For this review, use the dimensioned drawing (mm, ordinates from the lowest corner) and the shaded views. A direction names the side the tool comes from. Coordinates: 2 decimals unless noted, no trailing zeros. Loops run counter-clockwise (first coordinate to the right, second up) from the corner with the lowest first, then second, coordinate; pieces in that order, holes last. Notation, with made-up numbers: M 67,-39.5 L 77,-39.5 A24 ccw 77,-27.5 Z; hole C -38,-3 d11. An arc over 180 degrees is marked long. Use CSV: the item, a comma, the result in double quotes. Start each with the question number.
1. For L1, parallel to X at y = 1, z = 13; L2, parallel to Z at x = 12.75, y = 3.5; L3, parallel to Y at x = 13.75, z = 12.5, list the stretches that pass through material, from the lowest coordinate up.
2. Add section D-D, the plane y = 7.75. Write out the cut boundary in (x, z).
3. Add section B-B, the plane z = 9.75. Write out the cut boundary in (x, y).
4. Add section C-C, the plane x = 12.7. Write out the cut boundary in (y, z).
5. Clearance check with flat-ended pins moving along their axes: P1, Ø0.6, axis at y = 0.5, z = 19.5, coming from the -X side; P2, Ø5, axis at x = 11, y = 5.5, coming from the -Z side; P3, Ø0.6, axis at y = 0.5, z = 20.5, coming from the +X side; P4, Ø2, axis at y = 3, z = 11.5, coming from the -X side. State where each tip first meets the part, or that it passes through.
6. Add section A-A, the plane y = 0.5. Write out the cut boundary in (x, z), then the cut area to 3 significant figures.
7. Tool access review of the marked faces 1 and 2: name each direction out of +Z, -Z, +X, -X, +Y, -Y from which nothing blocks a thin tool from reaching the whole face with its end or side.
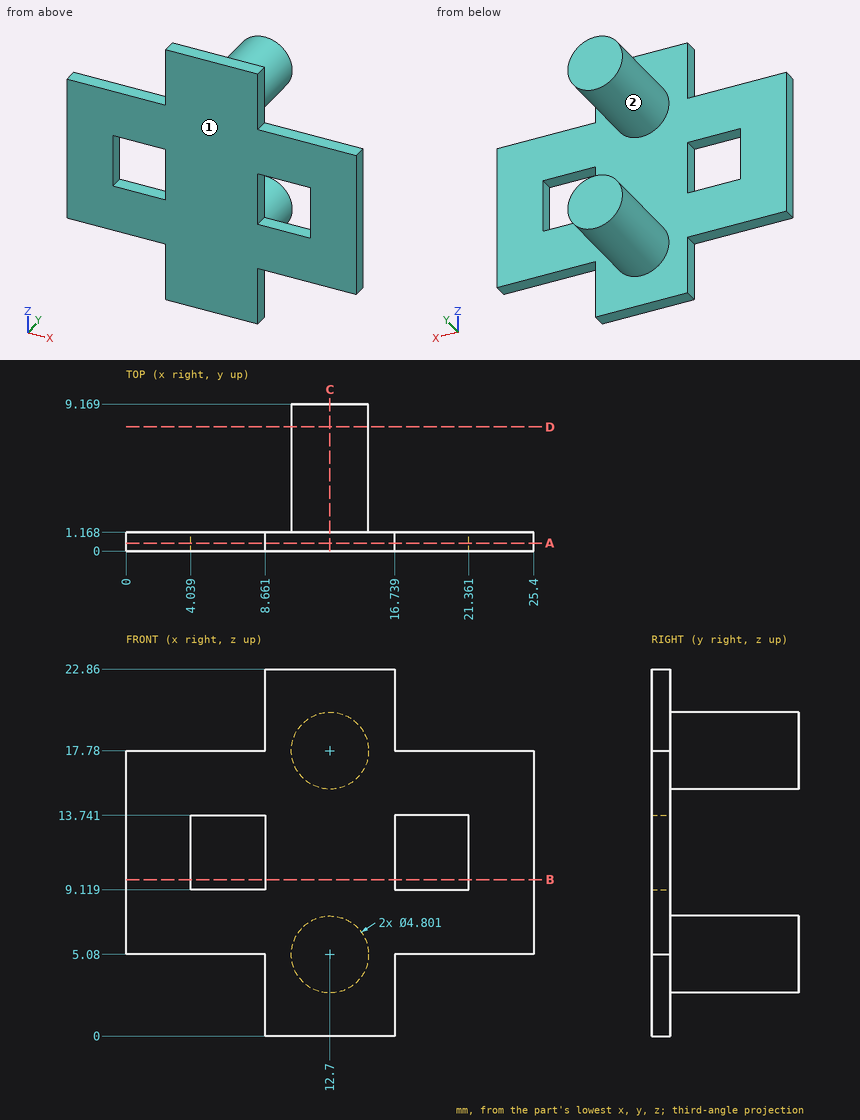
Computed:
1,L1,"x = 0 to 4.04, 8.66 to 16.74, 21.36 to 25.4"
1,L2,"z = 2.68 to 7.48, 15.38 to 20.18"
1,L3,"y = 0 to 1.17"
2,outline,"C 12.7,5.08 d4.8; C 12.7,17.78 d4.8"
3,outline,"M 0,0 L 4.04,0 L 4.04,1.17 L 0,1.17 Z; M 8.66,0 L 16.74,0 L 16.74,1.17 L 8.66,1.17 Z; M 21.36,0 L 25.4,0 L 25.4,1.17 L 21.36,1.17 Z"
4,outline,"M 0,0 L 1.17,0 L 1.17,2.68 L 9.17,2.68 L 9.17,7.48 L 1.17,7.48 L 1.17,15.38 L 9.17,15.38 L 9.17,20.18 L 1.17,20.18 L 1.17,22.86 L 0,22.86 Z"
5,P1,"stops at x = 8.66"
5,P2,"stops at z = 2.68"
5,P3,"stops at x = 16.74"
5,P4,"passes through"
6,outline,"M 0,5.08 L 8.66,5.08 L 8.66,0 L 16.74,0 L 16.74,5.08 L 25.4,5.08 L 25.4,17.78 L 16.74,17.78 L 16.74,22.86 L 8.66,22.86 L 8.66,17.78 L 0,17.78 Z; hole M 4.04,9.12 L 8.66,9.12 L 8.66,13.74 L 4.04,13.74 Z; hole M 16.74,9.12 L 21.36,9.12 L 21.36,13.74 L 16.74,13.74 Z"
6,area,"362 mm^2"
7,face 1,"+Z, -Z, +X, -X, -Y"
7,face 2,"+Y"
